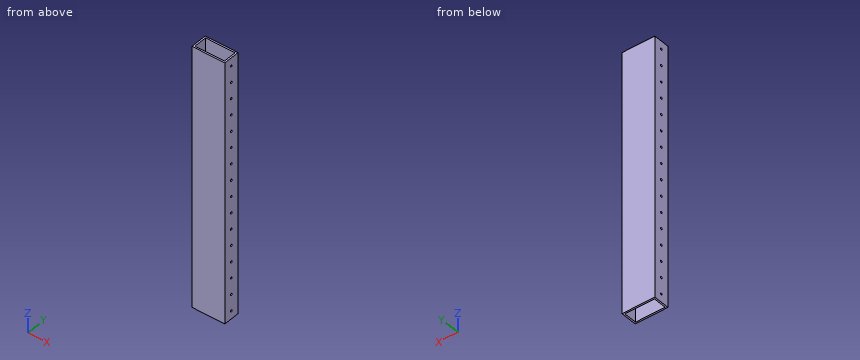
Autodesk Inventor part; units mm, degrees
ref_plane "YZ Plane" through (0, 0, 0) normal (1, 0, 0) x (0, 1, 0)
ref_plane "XZ Plane" through (0, 0, 0) normal (0, 1, 0) x (-1, 0, 0)
ref_plane "XY Plane" through (0, 0, 0) normal (0, 0, 1) x (1, 0, 0)
sketch "Sketch1" plane through (0, 0, 0) normal (0, 0, 1) x (1, 0, 0)
  line L0 (-25.4, 12.7) -> (25.4, 12.7)
  line L1 (25.4, 12.7) -> (25.4, -12.7)
  line L2 (25.4, -12.7) -> (-25.4, -12.7)
  line L3 (-25.4, -12.7) -> (-25.4, 12.7)
  line L4 (-25.4, 12.7) -> (25.4, -12.7) construction
  line L5 (25.4, 12.7) -> (-25.4, -12.7) construction
  line L6 (22.86, 10.16) -> (-22.86, 10.16)
  line L7 (-22.86, 10.16) -> (-22.86, -10.16)
  line L8 (-22.86, -10.16) -> (22.86, -10.16)
  line L9 (22.86, -10.16) -> (22.86, 10.16)
  point P0 (0, 0)
  dimension "d0" = 50.8
  dimension "d1" = 25.4
  dimension "d2" = 2.54
extrude "Extrusion1" add sketch "Sketch1" along normal blind 406.4
sketch "Sketch2" plane through (25.4, -12.7, 0) normal (1, 0, 0) x (0, 0, -1)
  circle A0 centre (-12.7, 12.7) radius 1.5875
  line L0 (0, 0) -> (0, 25.4)
  point P0 (0, 12.7)
  point P1 (0, 12.7)
  dimension "d5" = 3.175
  dimension "d6" = 12.7
extrude "Extrusion2" cut sketch "Sketch2" against normal through all
pattern_linear "Rectangular Pattern1" count 36 spacing 25.4 along (0, 0, 1) of "Extrusion2"
properties part number "rectangular tube-01"
For this review, take the finished solid that the model builds, in its own axes (mm). Coordinates: 2 decimals unless noted, no trailing zeros. Order: outer loops, then holes, each group sorted by start corner. A loop starts at its lowest first (then second) coordinate and runs counter-clockwise, first axis right, second up. Notation, with made-up numbers: (25, 61.5) -> (41, 61.5) arc R27 ccw to (41, 88.5) -> close; hole circle Ø1 at (83, 84). An arc over 180 degrees is marked (long way). Answer as CSV lines item,"result".
Q1. Wall thickness on line 1 along X through (y, z) = (-4.5, 166.5); line 2 along Y through (x, z) = (24.05, 342.9); line 3 along Y through (x, z) = (15, 110): over which ranges is each line inside the solid? List them lowest first. Write a range as [from, to].
Model answer:
line 1,"x = [-25.4, -22.86], [22.86, 25.4]"
line 2,"y = [-12.7, -1.59], [1.59, 12.7]"
line 3,"y = [-12.7, -10.16], [10.16, 12.7]"
Q2. We need section B-B (x = 16). State the section outline as (y, z) points, plus the area to 3 significant figures.
Model answer:
outline,"(-12.7, 0) -> (-10.16, 0) -> (-10.16, 406.4) -> (-12.7, 406.4) -> close; (10.16, 0) -> (12.7, 0) -> (12.7, 406.4) -> (10.16, 406.4) -> close"
area,"2,060 mm2"
Q3. We need section A-A (z = 74). State the section outline as (x, y) points.
Model answer:
outline,"(-25.4, -12.7) -> (25.4, -12.7) -> (25.4, 12.7) -> (-25.4, 12.7) -> close; hole (-22.86, -10.16) -> (22.86, -10.16) -> (22.86, 10.16) -> (-22.86, 10.16) -> close"
